For this review, take the finished solid that the model builds, in its own axes (mm). Round coordinates to 2 decimals unless told otherwise and drop trailing zeros. Write each loop counter-clockwise with the first axis right and the second up, starting at its lowest first coordinate (ties: lowest second). Pieces come first, ordered by that corner, then holes. Notation, with made-up numbers: M 87,61 L 121,61 A29 ccw 121,87 Z; hole C 42.25,8.5 d2. An arc over 180 degrees is marked long. Answer in a Markdown table with one row per item.
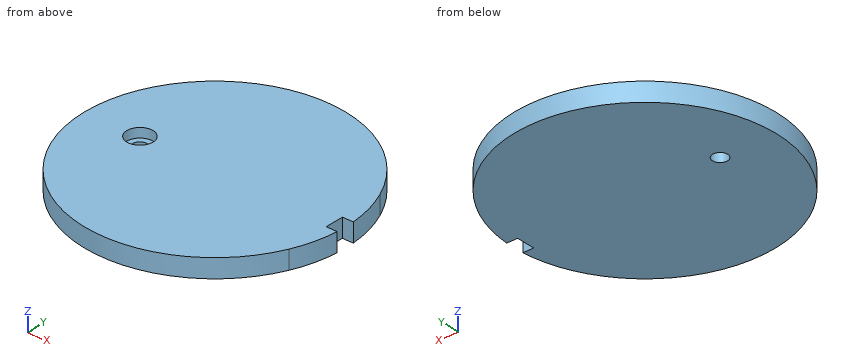
```python
from build123d import *

# Parameters (mm, degrees)
F0_R     = 3.5
F1_DEPTH = 5
F0_R_2   = 2
F2_DEPTH = 2.5


with BuildPart() as f1:
    # F0 (on Top) → F1 (new body)
    with BuildSketch(Plane.XY):
        with BuildLine():
            Line((31.788736, 2.5), (31.788736, 14.132672))
            ThreePointArc((31.788736, 14.132672), (-34.788736, 0), (31.788736, -14.132672))
            Line((31.788736, -14.132672), (31.788736, -2.5))
            Line((31.788736, -2.5), (31.788736, 2.5))
        make_face()
        with Locations((-20, 0)):
            Circle(F0_R, mode=Mode.SUBTRACT)
        with BuildLine():
            Line((31.788736, 2.5), (34.698792, 2.5))
            ThreePointArc((34.698792, 2.5), (33.748742, 8.442662), (31.788736, 14.132672))
            Line((31.788736, 14.132672), (31.788736, 2.5))
        make_face()
        with BuildLine():
            ThreePointArc((31.788736, -14.132672), (33.748742, -8.442662), (34.698792, -2.5))
            Line((34.698792, -2.5), (31.788736, -2.5))
            Line((31.788736, -2.5), (31.788736, -14.132672))
        make_face()
    extrude(amount=F1_DEPTH)

    # F0 (on Top) → F2 (join)
    with BuildSketch(Plane.XY):
        with Locations((-20, 0)):
            Circle(F0_R)
        with Locations((-20, 0)):
            Circle(F0_R_2, mode=Mode.SUBTRACT)
    extrude(amount=F2_DEPTH)


solid = f1.part
```
Q1. Take a section at A-A (y = 0). State the section outline as (x, z) points.
Found:
| item | result |
|---|---|
| outline | M -34.79,0 L -22,0 L -22,2.5 L -23.5,2.5 L -23.5,5 L -34.79,5 Z; M -18,0 L 31.79,0 L 31.79,5 L -16.5,5 L -16.5,2.5 L -18,2.5 Z |
Q2. Take a section at C-C (x = -20). State the section outline as (y, z) points (3 decimals), then the cut area to 3 significant figures.
Found:
| item | result |
|---|---|
| outline | M -28.465,0 L -2,0 L -2,2.5 L -3.5,2.5 L -3.5,5 L -28.465,5 Z; M 2,0 L 28.465,0 L 28.465,5 L 3.5,5 L 3.5,2.5 L 2,2.5 Z |
| area | 257 mm² |
Q3. Insertion check: P1, Ø5, axis at x = -20, y = 0, coming from the +Z side; P2, Ø2.5, axis at x = 33, z = 2, coming from the -Y side. Each pin has a flat end and moves straight along its axis. Give the tip position at first contact, or say it passes through.
Found:
| item | result |
|---|---|
| P1 | z = 2.5 |
| P2 | y = -14.22 |
Q4. For probe 1 along Y at (x, z) = (-20, 1.35) (3 decimals); probe 2 along X at (y, z) = (1, 4.3); probe 3 along Y at (x, z) = (-20, 3.1) (3 decimals), list the stretches that pass through material, from the lowest coordinate up.
Found:
| item | result |
|---|---|
| probe 1 | -28.465 to -2, 2 to 28.465 |
| probe 2 | -34.77 to -23.35, -16.65 to 31.79 |
| probe 3 | -28.465 to -3.5, 3.5 to 28.465 |
Q5. Take a section at D-D (y = -16.5). State the section outline as (x, z) points.
Found:
| item | result |
|---|---|
| outline | M -30.63,0 L 30.63,0 L 30.63,5 L -30.63,5 Z |
Q6. Take a section at B-B (z = 1.35). State the section outline as (x, y) points, then the cut area to 3 significant figures.
Found:
| item | result |
|---|---|
| outline | M 31.79,-14.13 A34.79 ccw 34.7,-2.5 L 31.79,-2.5 L 31.79,2.5 L 34.7,2.5 A34.79 ccw 31.79,14.13 A34.79 ccw long Z; hole C -20,0 d4 |
| area | 3,770 mm² |
